from build123d import *

# Parameters (mm, degrees)
SKETCH1_R           = 14
SKETCH1_R_2         = 2.25
BOSS_EXTRUDE1_DEPTH = 5
SKETCH2_R           = 1.5
CUT_EXTRUDE1_DEPTH  = 21.420577857
SKETCH4_R           = 3.5
CUT_EXTRUDE2_DEPTH  = 3
CIRPATTERN1_COUNT   = 2
SKETCH5_R           = 11.125
SKETCH5_R_2         = 6.125
BOSS_EXTRUDE2_DEPTH = 6
SKETCH6_R           = 3.5
CUT_EXTRUDE3_DEPTH  = 21.688160866
CHAMFER1_SIZE       = 3
FILLET1_START       = 5
FILLET1_DEPTH       = 7
SKETCH8_R           = 1.6
CUT_EXTRUDE4_DEPTH  = 23.649503429
CHAMFER2_SIZE       = 3
CIRPATTERN2_COUNT   = 2
CIRPATTERN2_ANGLE   = 100


with BuildPart() as part:
    # Sketch1 → Boss-Extrude1 (new body)
    with BuildSketch(Plane(origin=(0, 0, 0), x_dir=(1, 0, 0), z_dir=(0, 1, 0))):
        with Locations(Location((0, 0, 0), (0, 0, 270))):
            Circle(SKETCH1_R)
        with Locations(Location((0, 0, 0), (0, 0, 270))):
            Circle(SKETCH1_R_2, mode=Mode.SUBTRACT)
    extrude(amount=BOSS_EXTRUDE1_DEPTH)

    # Sketch2 → Cut-Extrude1 (cut, through all)
    with BuildSketch(Plane(origin=(0, 5, 0), x_dir=(1, 0, 0), z_dir=(0, 1, 0))):
        with Locations(Location((0, 9, 0), (0, 0, 270))):
            Circle(SKETCH2_R)
    cut_extrude1 = extrude(amount=-CUT_EXTRUDE1_DEPTH, mode=Mode.SUBTRACT)

    # Sketch4 → Cut-Extrude2 (cut)
    with BuildSketch(Plane(origin=(0, 5, 0), x_dir=(1, 0, 0), z_dir=(0, 1, 0))):
        with Locations(Location((0, 9, 0), (0, 0, 270))):
            Circle(SKETCH4_R)
    cut_extrude2 = extrude(amount=-CUT_EXTRUDE2_DEPTH, mode=Mode.SUBTRACT)

    # CirPattern1: Cut-Extrude1, Cut-Extrude2 ×2 about axis
    cirpattern1_axis = Axis((0, 0, 0), (0, 1, 0))
    add([cut_extrude1.rotate(cirpattern1_axis, i * 360 / CIRPATTERN1_COUNT) for i in range(1, CIRPATTERN1_COUNT)], mode=Mode.SUBTRACT)
    add([cut_extrude2.rotate(cirpattern1_axis, i * 360 / CIRPATTERN1_COUNT) for i in range(1, CIRPATTERN1_COUNT)], mode=Mode.SUBTRACT)

    # Sketch5 → Boss-Extrude2 (add)
    with BuildSketch(Plane(origin=(0, 5, 0), x_dir=(1, 0, 0), z_dir=(0, 1, 0))):
        with Locations(Location((0, 0, 0), (0, 0, 74.023861397))):
            Circle(SKETCH5_R)
        with Locations(Location((0, 0, 0), (0, 0, 105.450591775))):
            Circle(SKETCH5_R_2, mode=Mode.SUBTRACT)
    extrude(amount=BOSS_EXTRUDE2_DEPTH)

    # Sketch6 → Cut-Extrude3 (cut, through all)
    with BuildSketch(Plane(origin=(0, 5, 0), x_dir=(1, 0, 0), z_dir=(0, 1, 0))):
        with Locations(Location((0, 9, 0), (0, 0, 270))):
            Circle(SKETCH6_R)
        with Locations(Location((0, -9, 0), (0, 0, 331.028467776))):
            Circle(SKETCH6_R)
    extrude(amount=CUT_EXTRUDE3_DEPTH, mode=Mode.SUBTRACT)

    # Chamfer1
    # the kernel refuses this chamfer: 3 mm, written as the material it takes off along each edge
    with BuildSketch(Plane(origin=(0, 5, 0), x_dir=(0, 0, 1), z_dir=(-1, 0, 0))) as chamfer1_piece_1_section:
        Polygon((14, -CHAMFER1_SIZE), (14 - CHAMFER1_SIZE, 0), (14, 0), align=None)
    chamfer1_piece_1 = revolve(axis=Axis((0, 5, 0), (0, 1, 0)), mode=Mode.PRIVATE)
    chamfer1_piece_1 = chamfer1_piece_1 - Plane(origin=(0, 5, 0), x_dir=(0.2752370049355325, 0, -0.9613764044920791), z_dir=(0, -1, 0)) * Cylinder(11.125, 56, mode=Mode.PRIVATE)
    add(chamfer1_piece_1, mode=Mode.SUBTRACT)

    # Fillet1: read off the stored shape, not the designer's step
    # Fillet1 outline → Fillet1 (cut)
    with BuildSketch(Plane(origin=(0, 0, 0), x_dir=(1, 0, 0), z_dir=(0, 1, 0)).offset(FILLET1_START)):
        with BuildLine():
            ThreePointArc((2.73704056, -6.818576389), (2.537172315, -6.005807905), (3.025150093, -5.325794956))
            ThreePointArc((3.025150093, -5.325794956), (2.346304597, -5.65778046), (1.631744733, -5.903645833))
            ThreePointArc((1.631744733, -5.903645833), (2.231780839, -6.303863081), (2.73704056, -6.818576389))
        make_face()
        with BuildLine():
            ThreePointArc((1.631744733, 5.903645833), (2.346304597, 5.65778046), (3.025150093, 5.325794956))
            ThreePointArc((3.025150093, 5.325794956), (2.537172315, 6.005807905), (2.73704056, 6.818576389))
            ThreePointArc((2.73704056, 6.818576389), (2.231780839, 6.303863081), (1.631744733, 5.903645833))
        make_face()
        with BuildLine():
            ThreePointArc((-2.73704056, -6.818576389), (-2.231780839, -6.303863081), (-1.631744733, -5.903645833))
            ThreePointArc((-1.631744733, -5.903645833), (-2.346304597, -5.65778046), (-3.025150093, -5.325794956))
            ThreePointArc((-3.025150093, -5.325794956), (-2.537172315, -6.005807905), (-2.73704056, -6.818576389))
        make_face()
        with BuildLine():
            ThreePointArc((-3.025150093, 5.325794956), (-2.346304597, 5.65778046), (-1.631744733, 5.903645833))
            ThreePointArc((-1.631744733, 5.903645833), (-2.231780839, 6.303863081), (-2.73704056, 6.818576389))
            ThreePointArc((-2.73704056, 6.818576389), (-2.537172315, 6.005807905), (-3.025150093, 5.325794956))
        make_face()
    extrude(amount=FILLET1_DEPTH, mode=Mode.SUBTRACT)

    # Sketch8 → Cut-Extrude4 (cut, symmetric)
    with BuildSketch(Plane(origin=(0, 0, 0), x_dir=(0, -1, 0), z_dir=(-0.6427876096865406, 0, 0.7660444431189771))):
        with Locations(Location((-8.625, 0, 0), (0, 0, 90))):
            Circle(SKETCH8_R)
    cut_extrude4 = extrude(amount=CUT_EXTRUDE4_DEPTH, both=True, mode=Mode.SUBTRACT)

    # Chamfer2
    # the kernel refuses this chamfer: 3 mm, written as the material it takes off along each edge
    with BuildSketch(Plane(origin=(0, 11, 0), x_dir=(-0.4035609850169031, 0, 0.9149527481636345), z_dir=(-0.9149527481636345, 0, -0.4035609850169031))) as chamfer2_piece_1:
        Polygon((11.125, -CHAMFER2_SIZE), (11.125 - CHAMFER2_SIZE, 0), (11.125, 0), align=None)
    revolve(axis=Axis((0, 11, 0), (0, 1, 0)), revolution_arc=227.60196489, mode=Mode.SUBTRACT)
    with BuildSketch(Plane(origin=(0, 11, 0), x_dir=(0.40356098501590637, 0, -0.914952748164074), z_dir=(0.914952748164074, 0, 0.40356098501590637))) as chamfer2_piece_2:
        Polygon((11.125, -CHAMFER2_SIZE), (11.125 - CHAMFER2_SIZE, 0), (11.125, 0), align=None)
    revolve(axis=Axis((0, 11, 0), (0, 1, 0)), revolution_arc=227.60196489, mode=Mode.SUBTRACT)

    # CirPattern2: Cut-Extrude4 ×2 about axis
    cirpattern2_axis = Axis((0, 5, 0), (0, -1, 0))
    for i in range(1, CIRPATTERN2_COUNT):
        add(cut_extrude4.rotate(cirpattern2_axis, i * CIRPATTERN2_ANGLE / (CIRPATTERN2_COUNT - 1)), mode=Mode.SUBTRACT)


solid = part.part
The listing builds one solid part. Answer for the finished solid, in the listing's coordinates (mm). A direction names the side the tool comes from. Coordinates: 2 decimals unless noted, no trailing zeros. Write each loop counter-clockwise with the first axis right and the second up, starting at its lowest first coordinate (ties: lowest second). Pieces come first, ordered by that corner, then holes. Notation, with made-up numbers: (85.5, -39.75) - (104.5, -39.75) arc R26 ccw to (104.5, -2.75) - close; hole circle Ø2 at (-4.5, 67.5). An arc over 180 degrees is marked (long way). Return JSON: item names as keys, results as strings.
1. The part is cut by section B-B on z = 0. Determine the outline of the cut face in (x, y) (3 decimals).
Final values:
{"outline": "(-14, 0) - (-2.25, 0) - (-2.25, 5) - (-6.125, 5) - (-6.125, 11) - (-8.125, 11) - (-11.125, 8) - (-11.125, 4.875) - (-14, 2) - close; (2.25, 0) - (14, 0) - (14, 2) - (11.125, 4.875) - (11.125, 8) - (8.125, 11) - (6.125, 11) - (6.125, 5) - (2.25, 5) - close"}
2. The part is cut by section C-C on y = 9. Count the separate pieces of the cut face and the enclosed holes in it, then the cut area to 3 significant figures.
Final values:
{"separate pieces": "6", "enclosed holes": "0", "area": "104 mm^2"}
3. The part is cut by section D-D on y = 1.5. Determine the outline of the cut face in (x, z), then the cut area to 3 significant figures.
Final values:
{"outline": "circle Ø28 at (0, 0); hole circle Ø4.5 at (0, 0); hole circle Ø3 at (0, -9); hole circle Ø3 at (0, 9)", "area": "586 mm^2"}
4. Which of the six approach directions +Z, -Z, +X, -X, +Y, -Y give full straight-line access (tool end or side, diameter ignored) to faces 1 (the face through (5.346, 7.063, 5.832)), 2 (the face through (2.54, 7.96, -5.99))?
Final values:
{"face 1": "none", "face 2": "+Y"}
5. For a pull along Z with two mould halves and no side action, classify faces 3 (the face through (3.38, 4.74, 10.74)), 4 (the face through (0.07, 1.01, -10.5)), 5 (the face through (6.3, 11, -0.2)) as +Z half, -Z half, draft (parallel to the pull), parting line (faces both ways), or undercut.
Final values:
{"face 3": "parting line", "face 4": "undercut", "face 5": "draft"}
6. Consider line 1 along X through (y, z) = (1.95, 0); line 2 along Y through (x, z) = (0.25, 3.25); line 3 along Z through (x, y) = (3, 2.75). Determine where each line is inside the solid, lowest interval first.
Final values:
{"line 1": "-14 to -2.25, 2.25 to 14", "line 2": "0 to 5", "line 3": "-12.91 to -10.8, -7.2 to 7.2, 10.8 to 12.91"}
7. The part is cut by section A-A on y = 6.5. Determine the outline of the cut face in (x, z) (3 decimals), then the cut area to 3 significant figures.
Final values:
{"outline": "(-3.062, -10.695) arc R3.5 cw to (-2.737, -6.819) arc R1 ccw to (-3.025, -5.326) arc R6.125 cw to (-3.025, 5.326) arc R1 ccw to (-2.737, 6.819) arc R3.5 cw to (-3.062, 10.695) arc R11.125 ccw to start; (2.737, -6.819) arc R3.5 cw to (3.062, -10.695) arc R11.125 ccw to (3.062, 10.695) arc R3.5 cw to (2.737, 6.819) arc R1 ccw to (3.025, 5.326) arc R6.125 cw to (3.025, -5.326) arc R1 ccw to start", "area": "207 mm^2"}
8. Each of these flat-tipped pins is pushed along its axis until it touches: pin 1 Ø0.7 at (x, z) = (-2, -6) entering from +Y; pin 2 Ø1 at (x, y) = (3.5, 3.5) entering from -Z; pin 3 Ø2.5 at (x, z) = (0, 0) entering from -Y; pin 4 Ø3.5 at (x, z) = (0, -9) entering from +Y. Where does it stop, or does it pass through?
Final values:
{"pin 1": "y = 5", "pin 2": "z = -12.54", "pin 3": "through", "pin 4": "y = 2"}
